Here's how the part is built. I have some questions about the finished solid (model axes, mm). A direction names the side the tool comes from. Round coordinates to 2 decimals unless told otherwise and drop trailing zeros. Write each loop counter-clockwise with the first axis right and the second up, starting at its lowest first coordinate (ties: lowest second). Pieces come first, ordered by that corner, then holes. Notation, with made-up numbers: (8, -29.75) -> (41, -29.75) arc R15 cw to (41, -5.75) -> close; hole circle Ø5 at (-4.75, 14.25). An arc over 180 degrees is marked (long way). Answer as CSV lines item,"result".
```python
from build123d import *

# Parameters (mm, degrees)
F2_R = 2


# Not quite as in the source:
# - a fillet or chamfer that OpenCascade refuses, or shapes differently, is made with other operations: its cross-section is extruded or revolved along the edge and cut away or added


with BuildPart() as f1:
    # F0 (on Front) → F1 (revolve)
    with BuildSketch(Plane.XZ):
        Polygon((15.8820929868, -20), (15.8820929868, 0), (15.8820929868, 20), (25, 30.8662984399), (23.9358222275, 30.8662984399), (14.5927630612, 20.7279404685), (14.5927630612, 0.3639702343), (14.5927630612, -20), (21.0905159717, -28.2129982056), (2.4876487441, -28.2129982056), (2.4876487441, -29.5023282056), (22.5661631538, -29.5023282056), (23.8554930795, -29.5023282056), align=None)
    revolve(axis=Axis((0, 0, 0), (0, 0, -1)))

    # F2
    f2_edges = [f1.edges().sort_by_distance(p)[0] for p in [
        (-15.882093, 0, -20),
        (-15.882093, 0, 20),
        (-23.855493, 0, -29.502328),
    ]]
    fillet(f2_edges, radius=F2_R)

    # F3: fillet of radius 1.5 on 1 edges, made by hand

    # F3_s1 → F3_t2 (revolve, cut)
    with BuildSketch(Plane.XZ):
        with BuildLine():
            ThreePointArc((23.7026404335, 29.319932157), (24.0367869093, 30.060330686), (23.9359604662, 30.8663566642))
            Line((23.9359604662, 30.8663566642), (23.9636082001, 30.878001526))
            ThreePointArc((23.9636082001, 30.878001526), (24.4679802331, 30.8962984399), (25, 30.8962984399))
            Line((25, 30.8962984399), (25.0229813333, 30.8470148116))
            ThreePointArc((25.0229813333, 30.8470148116), (24.3742440967, 30.0738798792), (23.7256217668, 29.3006485287))
            Line((23.7256217668, 29.3006485287), (23.7026404335, 29.319932157))
        make_face()
    revolve(axis=Axis((0, 0, 30.8662984399), (0, 0, -1)), mode=Mode.SUBTRACT)


solid = f1.part
```
1. If we mould it in two halves opening along Y, with no side actions, what happens to faces 1 (the face through (-4, 0, -29.502)), 2 (the face through (16.035, -5.05, 21.107)), 3 (the face through (4, 0, -28.213))? For each: released by +Y, released by -Y, zero draft, split by the parting line, or undercut.
Numbers:
face 1,"zero draft"
face 2,"split by the parting line"
face 3,"undercut"
2. Suppose I cut it at C-C on z = 21.5. Please give me the cut outline in (x, y), and give its area (3 significant figures).
Numbers:
outline,"circle Ø34.28 at (0, 0); hole circle Ø30.61 at (0, 0)"
area,"187 mm^2"
3. For pin 1 Ø8 at (x, y) = (1, 10) entering from +Z; pin 2 Ø10 at (y, z) = (-4, 6) entering from +X; pin 3 Ø1.5 at (x, y) = (8.5, 11) entering from +Z, each with a flat end and sliding along its axis, tell me the tip position at first contact or that it passes through.
Numbers:
pin 1,"stops at z = -28.21"
pin 2,"stops at x = 15.88"
pin 3,"stops at z = 20.79"
4. Suppose I cut it at A-A on z = 15. Please give me the cut outline in (x, y).
Numbers:
outline,"circle Ø31.76 at (0, 0); hole circle Ø29.19 at (0, 0)"
5. If I drill on line 1 (X direction, y = 0, z = -10); line 2 (Z direction, x = 5, y = -8), over which ranges is the centre line in solid material (lowest first)?
Numbers:
line 1,"x = -15.88 to -14.59, 14.59 to 15.88"
line 2,"z = -29.5 to -28.21"
6. On a 3-axis mill with a long thin cutter (end or side, diameter ignored), from which of +Z, -Z, +X, -X, +Y, -Y can I reach the whole of each face in a straight line? I mean faces 4 (the face through (2.37, -0.75, -28.87)), 5 (the face through (-3.163, 14.246, 0.079)), 6 (the face through (15.815, -4.98, -20.832)). Say none if no direction works.
Numbers:
face 4,"+Z, -Z"
face 5,"+Z"
face 6,"none"
7. Suppose I cut it at B-B on y = -18. Count the separate pieces of the cut face and the enclosed holes in it, and give its area (3 significant figures).
Numbers:
separate pieces,"2"
enclosed holes,"1"
area,"124 mm^2"
